from build123d import *

# Parameters (mm, degrees)
SKETCH63_W                     = 76.2
SKETCH63_H                     = 101.6
BRACKET_INTERFACE_DEPTH        = 1.5
SKETCH57_R                     = 2.8
SKETCH57_R_2                   = 1.5
SKETCH57_R_3                   = 5
CUT_EXTRUDE7_DEPTH             = 2.54
STEPPER_FLANGE_STRIP_W         = 9
STEPPER_FLANGE_STRIP_H         = 1.5
STEPPER_FLANGE_STRIP_CUT_DEPTH = 76.2
STEPPER_FLANGE_DEPTH           = 76.2
BARREL_FLANGE_STRIP_W          = 9
BARREL_FLANGE_STRIP_H          = 1.5
BARREL_FLANGE_STRIP_CUT_DEPTH  = 76.2
BARREL_FLANGE_DEPTH            = 76.2
SKETCH75_R                     = 1.75
SKETCH75_R_2                   = 12.5
NEMA_17_PATTERN_DEPTH          = 2.54
SKETCH82_R                     = 27.305
CUT_EXTRUDE8_DEPTH             = 5
CUT_EXTRUDE17_REACH            = 136.904
CUT_EXTRUDE18_REACH            = 136.904
SKETCH145_R                    = 2.667


# Sheet-metal steps are written as plain solids
with BuildPart() as part:
    # Sketch63 → Bracket_Interface (new body)
    with BuildSketch(Plane(origin=(0, 0, 0), x_dir=(0, 0, -1), z_dir=(1, 0, 0))):
        Rectangle(SKETCH63_W, SKETCH63_H)
    extrude(amount=-BRACKET_INTERFACE_DEPTH)

    # Sketch57 → Cut-Extrude7 (cut)
    # profile 1 of 7: a face of its own
    with BuildSketch(Plane(origin=(0, 0, 0), x_dir=(0, 0, -1), z_dir=(1, 0, 0))):
        with Locations((9.203487694, 8.439536918)):
            Circle(SKETCH57_R)
        with Locations((9.203487694, 8.439536918)):
            Circle(SKETCH57_R_2, mode=Mode.SUBTRACT)
    # profile 2 of 7: a face of its own
    with BuildSketch(Plane(origin=(0, 0, 0), x_dir=(0, 0, -1), z_dir=(1, 0, 0))):
        with Locations((23.203487694, 8.439536918)):
            Circle(SKETCH57_R)
        with Locations((23.203487694, 8.439536918)):
            Circle(SKETCH57_R_2, mode=Mode.SUBTRACT)
    # profile 3 of 7: a face of its own
    with BuildSketch(Plane(origin=(0, 0, 0), x_dir=(0, 0, -1), z_dir=(1, 0, 0))):
        with Locations((0, -19.210463082)):
            Circle(SKETCH57_R_3)
    # profile 4 of 7: a face of its own
    with BuildSketch(Plane(origin=(0, 0, 0), x_dir=(0, 0, -1), z_dir=(1, 0, 0))):
        with Locations((-19.296512306, -0.360463082)):
            Circle(SKETCH57_R_2)
    # profile 5 of 7: a face of its own
    with BuildSketch(Plane(origin=(0, 0, 0), x_dir=(0, 0, -1), z_dir=(1, 0, 0))):
        with Locations((-1.796512306, 18.539536918)):
            Circle(SKETCH57_R_2)
    # profile 6 of 7: a face of its own
    with BuildSketch(Plane(origin=(0, 0, 0), x_dir=(0, 0, -1), z_dir=(1, 0, 0))):
        with Locations((19.703487694, 20.989536918)):
            Circle(SKETCH57_R_3)
    # profile 7 of 7: a face of its own
    with BuildSketch(Plane(origin=(0, 0, 0), x_dir=(0, 0, -1), z_dir=(1, 0, 0))):
        with Locations((-20.296512306, 20.989536918)):
            Circle(SKETCH57_R_3)
    extrude(amount=-CUT_EXTRUDE7_DEPTH, mode=Mode.SUBTRACT)


with BuildPart() as body_2:
    # of the pieces the cut leaves, the one that is kept (cut_extrude7_keep)
    add(part.part.solids().sort_by_distance((0, 50.8, 38.1))[0])

    # Stepper_Flange strip (across the edge) → Stepper_Flange strip cut (cut)
    with BuildSketch(Plane(origin=(0, 50.8, -38.1), x_dir=(0, -1, 0), z_dir=(0, 0, 1))):
        with Locations((-3, -0.75)):
            Rectangle(STEPPER_FLANGE_STRIP_W, STEPPER_FLANGE_STRIP_H)
    extrude(amount=STEPPER_FLANGE_STRIP_CUT_DEPTH, mode=Mode.SUBTRACT)

    # Stepper_Flange section (across the edge) → Stepper_Flange (add)
    with BuildSketch(Plane(origin=(0, 50.8, -38.1), x_dir=(0, -1, 0), z_dir=(0, 0, 1))):
        with BuildLine():
            Line((-1.5, 1.5), (-1.5, 66.04))
            Line((-1.5, 66.04), (0, 66.04))
            Line((0, 66.04), (0, 1.5))
            ThreePointArc((0, 1.5), (0.439339828, 0.439339828), (1.5, 0))
            Line((1.5, 0), (1.5, -1.5))
            ThreePointArc((1.5, -1.5), (-0.621320344, -0.621320344), (-1.5, 1.5))
        make_face()
    extrude(amount=STEPPER_FLANGE_DEPTH)

    # Barrel_Flange strip (across the edge) → Barrel_Flange strip cut (cut)
    with BuildSketch(Plane(origin=(0, -50.8, 38.1), x_dir=(0, 1, 0), z_dir=(0, 0, -1))):
        with Locations((-3, -0.75)):
            Rectangle(BARREL_FLANGE_STRIP_W, BARREL_FLANGE_STRIP_H)
    extrude(amount=BARREL_FLANGE_STRIP_CUT_DEPTH, mode=Mode.SUBTRACT)

    # Barrel_Flange section (across the edge) → Barrel_Flange (add)
    with BuildSketch(Plane(origin=(0, -50.8, 38.1), x_dir=(0, 1, 0), z_dir=(0, 0, -1))):
        with BuildLine():
            Line((-1.5, 1.5), (-1.5, 76.2))
            Line((-1.5, 76.2), (0, 76.2))
            Line((0, 76.2), (0, 1.5))
            ThreePointArc((0, 1.5), (0.439339828, 0.439339828), (1.5, 0))
            Line((1.5, 0), (1.5, -1.5))
            ThreePointArc((1.5, -1.5), (-0.621320344, -0.621320344), (-1.5, 1.5))
        make_face()
    extrude(amount=BARREL_FLANGE_DEPTH)

    # Sketch75 → NEMA_17_Pattern (cut)
    with BuildSketch(Plane(origin=(0, 52.3, 0), x_dir=(1, 0, 0), z_dir=(0, 1, 0))):
        with Locations(Location((23.04, 15.5, 0), (0, 0, 180))):
            Circle(SKETCH75_R)
        with Locations(Location((54.04, 15.5, 0), (0, 0, 180))):
            Circle(SKETCH75_R)
        with Locations(Location((54.04, -15.5, 0), (0, 0, 180))):
            Circle(SKETCH75_R)
        with Locations(Location((23.04, -15.5, 0), (0, 0, 180))):
            Circle(SKETCH75_R)
        with Locations(Location((38.54, 0, 0), (0, 0, 180))):
            Circle(SKETCH75_R_2)
    extrude(amount=-NEMA_17_PATTERN_DEPTH, mode=Mode.SUBTRACT)

    # Sketch82 → Cut-Extrude8 (cut)
    with BuildSketch(Plane(origin=(0, -50.8, 0), x_dir=(1, 0, 0), z_dir=(0, 1, 0))):
        with Locations(Location((38.54, 0, 0), (0, 0, 180))):
            Circle(SKETCH82_R)
    extrude(amount=-CUT_EXTRUDE8_DEPTH, mode=Mode.SUBTRACT)

    # Sketch142 → Cut-Extrude17 (cut, up to next)
    with BuildSketch(Plane.XZ.offset(52.3), mode=Mode.PRIVATE) as cut_extrude17_sk1:
        with BuildLine():
            Line((19.363, 19.437224493), (19.363, 27.94))
            Line((19.363, 27.94), (57.717, 27.94))
            Line((57.717, 27.94), (57.717, 19.437224493))
            ThreePointArc((57.717, 19.437224493), (38.54, 27.305), (19.363, 19.437224493))
        make_face()
    cut_extrude17_tool1 = extrude(cut_extrude17_sk1.sketch, amount=-CUT_EXTRUDE17_REACH, mode=Mode.PRIVATE) & body_2.part
    cut_extrude17 = cut_extrude17_tool1.solids().sort_by_distance((38.54, -52.3, 27.697852))[0]
    add(cut_extrude17, mode=Mode.SUBTRACT)

    # Mirror1: Cut-Extrude17 across plane
    add(cut_extrude17.mirror(Plane.XY), mode=Mode.SUBTRACT)

    # Sketch145 → Cut-Extrude18 (cut, up to next)
    with BuildSketch(Plane(origin=(0, 52.3, 0), x_dir=(1, 0, 0), z_dir=(0, 1, 0)), mode=Mode.PRIVATE) as cut_extrude18_sk1:
        with Locations(Location((38.54, 28.410128662, 0), (0, 0, 180))):
            Circle(SKETCH145_R)
    cut_extrude18_tool1 = extrude(cut_extrude18_sk1.sketch, amount=-CUT_EXTRUDE18_REACH, mode=Mode.PRIVATE) & body_2.part
    # Sketch145 → Cut-Extrude18 (cut, up to next)
    with BuildSketch(Plane(origin=(0, 52.3, 0), x_dir=(1, 0, 0), z_dir=(0, 1, 0)), mode=Mode.PRIVATE) as cut_extrude18_sk2:
        with Locations(Location((38.54, -29.364200147, 0), (0, 0, 180))):
            Circle(SKETCH145_R)
    cut_extrude18_tool2 = extrude(cut_extrude18_sk2.sketch, amount=-CUT_EXTRUDE18_REACH, mode=Mode.PRIVATE) & body_2.part
    add(cut_extrude18_tool1.solids().sort_by_distance((38.54, 52.3, -28.410129))[0], mode=Mode.SUBTRACT)
    add(cut_extrude18_tool2.solids().sort_by_distance((38.54, 52.3, 29.3642))[0], mode=Mode.SUBTRACT)


solid = body_2.part
Verification items for the finished model (mm, model axes). A direction names the side the tool comes from. Give positions to 0.01 mm unless a question says otherwise; leave off trailing zeros. Order: outer loops, then holes, each group sorted by start corner. A loop starts at its lowest first (then second) coordinate and runs counter-clockwise, first axis right, second up. Notation, with made-up numbers: M 0.5,-1 L 39.5,-1 A14 cw 39.5,22 Z; hole C -11,24.5 d4. An arc over 180 degrees is marked long. Use one line per item in the form item = value. Start each with the question number.
Q1. Section check D-D (z = -32.5). Enter the section's corners in (x, y), then the cut area to 3 significant figures.
Q2. Scan lines: line 1 along Z through (x, y) = (54, 51); line 2 along X through (y, z) = (-31, -5.5); line 3 along Y through (x, z) = (31, -11.5). Record each from-to range of solid material in increasing order. Write a range as [from, to].
Q3. Section check C-C (x = 64.5). Enter the section's corners in (y, z).
Q4. Section check B-B (x = 38.54). Enter the section's corners in (y, z).
Q5. Go/stop test with flat-tipped pins: pin 1 Ø4.5 at (x, z) = (38.54, 29.36) entering from +Y; pin 2 Ø4 at (y, z) = (-24.5, -13.5) entering from +X; pin 3 Ø4.5 at (x, z) = (54.04, 15.5) entering from +Y; pin 4 Ø5.5 at (x, z) = (23.04, -15.5) entering from -Y. Record where each tip stops, or that it passes through.
Q6. Section check A-A (x = 23.04). Enter the section's corners in (y, z).
Q7. Mould release check, pull along Y, two halves, no side actions. Record for faces 6 (the cylindrical face through (23.268, 51.56, -13.765)), 7 (the cylindrical face through (-0.74, 24.37, -16.02)), 8 (the cylindrical face through (-0.64, -51.4, 0.53)): +Y half, -Y half, draft (parallel to the pull), parting line (faces both ways), or undercut.
Q8. Access from +Z, -Z, +X, -X, +Y, -Y to the whole of each face (thin tool, end or side, straight path). Record for faces 1 (the flat face through (63, -52.3, 17)), 2 (the cylindrical face through (23.268, 51.56, 17.235)), 3 (the flat face through (0, 1, 1)), 4 (the cylindrical face through (11.237, -51.54, -0.303)), 5 (the cylindrical face through (40.5, 51.6, -26.6)).
Evaluation:
q1.outline = M -1.5,-49.3 A3 ccw 1.5,-52.3 L 76.2,-52.3 L 76.2,-50.8 L 1.5,-50.8 A1.5 cw 0,-49.3 L 0,49.3 A1.5 cw 1.5,50.8 L 66.04,50.8 L 66.04,52.3 L 1.5,52.3 A3 ccw -1.5,49.3 Z
q1.area = 367 mm2
q2.line_1 = [-38.1, -17.25], [-13.75, 13.75], [17.25, 38.1]
q2.line_2 = [-1.5, 0]
q2.line_3 = [50.8, 52.3]
q3.outline = M -52.3,-38.1 L -50.8,-38.1 L -50.8,-8.46 L -52.3,-8.46 Z; M -52.3,8.46 L -50.8,8.46 L -50.8,38.1 L -52.3,38.1 Z; M 50.8,-38.1 L 52.3,-38.1 L 52.3,38.1 L 50.8,38.1 Z
q4.outline = M -52.3,-38.1 L -50.8,-38.1 L -50.8,-27.94 L -52.3,-27.94 Z; M -52.3,27.94 L -50.8,27.94 L -50.8,38.1 L -52.3,38.1 Z; M 50.8,-38.1 L 52.3,-38.1 L 52.3,-31.08 L 50.8,-31.08 Z; M 50.8,-25.74 L 52.3,-25.74 L 52.3,-12.5 L 50.8,-12.5 Z; M 50.8,12.5 L 52.3,12.5 L 52.3,26.7 L 50.8,26.7 Z; M 50.8,32.03 L 52.3,32.03 L 52.3,38.1 L 50.8,38.1 Z
q5.pin_1 = -50.8
q5.pin_2 = 0
q5.pin_3 = 52.3
q5.pin_4 = 50.8
q6.outline = M -52.3,-38.1 L -50.8,-38.1 L -50.8,-27.94 L -52.3,-27.94 Z; M -52.3,27.94 L -50.8,27.94 L -50.8,38.1 L -52.3,38.1 Z; M 50.8,-38.1 L 52.3,-38.1 L 52.3,-17.25 L 50.8,-17.25 Z; M 50.8,-13.75 L 52.3,-13.75 L 52.3,13.75 L 50.8,13.75 Z; M 50.8,17.25 L 52.3,17.25 L 52.3,38.1 L 50.8,38.1 Z
q7.face_6 = draft
q7.face_7 = undercut
q7.face_8 = -Y half
q8.face_1 = +Z, -Z, +X, -X, -Y
q8.face_2 = +Y, -Y
q8.face_3 = +Z, -Z, +X
q8.face_4 = -Y
q8.face_5 = +Y
